Geometry check sheet. Reference: the model listing, model coordinates, mm. A direction names the side the tool comes from. Round coordinates to 2 decimals unless told otherwise and drop trailing zeros. Order: outer loops, then holes, each group sorted by start corner. A loop starts at its lowest first (then second) coordinate and runs counter-clockwise, first axis right, second up.
(1) Cross-section at B-B on y = -90.5. Enter the section's corners in (x, z).
(2) Cross-section at A-A on z = 0. Count the separate pieces of the cut face and the enclosed holes in it, and give its area (3 significant figures).
(3) Cross-section at C-C on x = 8.5. Enter the section's corners in (y, z).
(4) Draft check along Z on faces 3 (the face through (-11.942, -68, 94)), 4 (the face through (1.647, -98.101, -23.183)), 5 (the face through (-24.82, 16.948, -35.166)). Enter one of: pulls with the +Z half, pulls with the -Z half, needs draft (parallel to the pull), parting line crosses it, or undercut.
(5) Cross-section at D-D on z = 23. Enter the section's corners in (x, y).
(6) Set-up check for faces 1 (the face through (1.6, -150.4, 0.8)), 2 (the face through (-37.342, -67, 94)): record each of +Z, -Z, +X, -X, +Y, -Y from which the full face is reachable in a straight line by a thin tool's end or side.
(7) Thickness scan on L1, parallel to X at y = -138, z = -65.5; L2, parallel to Z at x = 10, y = -67; L3, parallel to Y at x = -18.5, z = 16. Record the ranges inside material, lowest first.
(8) Gauge pin test, flat ends, axial feed: P1, Ø3, axis at x = 13.5, y = -82, coming from the -Z side; P2, Ø4, axis at y = 2.5, z = 15, coming from the -X side; P3, Ø8, axis at x = 25, y = -57.5, coming from the -Z side; P4, Ø2, axis at x = -18, y = -28.5, coming from the +Z side. Record the tip position at first contact, or that the pin passes through.
from build123d import *

# Parameters (mm, degrees)
F2_R     = 19.05
F3_DEPTH = 127


with BuildPart() as f1:
    # F0 (on Top) → F1 (revolve)
    with BuildSketch(Plane.XY):
        Polygon((-37.342314, 46.434332), (-62.742314, 46.434332), (-62.742314, -29.765668), (64.257686, -29.765668), (64.257686, 46.434332), (38.857686, 46.434332), (38.857686, 23.949085), (13.457686, 23.949085), (13.457686, 46.434332), (-11.942314, 46.434332), (-11.942314, 23.949085), (-37.342314, 23.949085), align=None)
    revolve(axis=Axis((0.757686, -67.865668, 0), (1, 0, 0)))

    # F2 (on face) → F3 (cut, through all)
    with BuildSketch(Plane.YZ.offset(64.257686)):
        with BuildLine():
            ThreePointArc((-67.865668, 44.45), (-54.395284, 50.029616), (-48.815668, 63.5))
            ThreePointArc((-48.815668, 63.5), (-81.336052, 76.970384), (-67.865668, 44.45))
        make_face()
        with Locations((-131.365668, 0)):
            Circle(F2_R)
        with BuildLine():
            ThreePointArc((-67.865668, -44.45), (-81.336052, -76.970384), (-48.815668, -63.5))
            ThreePointArc((-48.815668, -63.5), (-54.395284, -50.029616), (-67.865668, -44.45))
        make_face()
        with BuildLine():
            ThreePointArc((-23.415668, 0), (-4.365668, -19.05), (14.684332, 0))
            ThreePointArc((14.684332, 0), (-4.365668, 19.05), (-23.415668, 0))
        make_face()
    extrude(amount=-F3_DEPTH, mode=Mode.SUBTRACT)


solid = f1.part
Found:
1. outline: (-62.74, -112.04) - (-37.34, -112.04) - (-37.34, -88.98) - (-11.94, -88.98) - (-11.94, -112.04) - (13.46, -112.04) - (13.46, -88.98) - (38.86, -88.98) - (38.86, -112.04) - (64.26, -112.04) - (64.26, -30.65) - (-62.74, -30.65) - close; (-62.74, 30.65) - (64.26, 30.65) - (64.26, 112.04) - (38.86, 112.04) - (38.86, 88.98) - (13.46, 88.98) - (13.46, 112.04) - (-11.94, 112.04) - (-11.94, 88.98) - (-37.34, 88.98) - (-37.34, 112.04) - (-62.74, 112.04) - close
2. separate pieces: 4
2. enclosed holes: 0
2. area: 7,390 mm2
3. outline: circle Ø228.6 at (-67.87, 0); hole circle Ø38.1 at (-131.37, 0); hole circle Ø76.2 at (-67.87, 0); hole circle Ø38.1 at (-67.87, -63.5); hole circle Ø38.1 at (-67.87, 63.5); hole circle Ø38.1 at (-4.37, 0)
4. face 3: needs draft
4. face 4: undercut
4. face 5: parting line crosses it
5. outline: (-62.74, -179.83) - (-37.34, -179.83) - (-37.34, -156.75) - (-11.94, -156.75) - (-11.94, -179.83) - (13.46, -179.83) - (13.46, -156.75) - (38.86, -156.75) - (38.86, -179.83) - (64.26, -179.83) - (64.26, -98.24) - (-62.74, -98.24) - close; (-62.74, -37.49) - (64.26, -37.49) - (64.26, 44.1) - (38.86, 44.1) - (38.86, 21.02) - (13.46, 21.02) - (13.46, 44.1) - (-11.94, 44.1) - (-11.94, 21.02) - (-37.34, 21.02) - (-37.34, 44.1) - (-62.74, 44.1) - close
6. face 1: +X, -X
6. face 2: none
7. L1: x = -62.74 to -37.34, -11.94 to 13.46, 38.86 to 64.26
7. L2: z = -114.3 to -82.53, -44.47 to -38.09, 38.09 to 44.47, 82.53 to 114.3
7. L3: y = -158.28 to -141.71, -121.03 to -102.44, -33.29 to -14.71, 5.97 to 22.54
8. P1: stops at z = -113.6
8. P2: passes through
8. P3: stops at z = -91.59
8. P4: stops at z = 83.41
